Could you check a few things on this drawing? It's one solid part, dimensions in mm from its lowest x, y, z. Give positions to 0.01 mm unless a question says otherwise; leave off trailing zeros. Order: outer loops, then holes, each group sorted by start corner. A loop starts at its lowest first (then second) coordinate and runs counter-clockwise, first axis right, second up. Notation, with made-up numbers: (32.25, 26.25) -> (52.25, 26.25) arc R28 ccw to (52.25, 53.25) -> close; hole circle Ø3 at (72, 45.25). An arc over 180 degrees is marked (long way). Write each question's results on one line, items separated by ' | '. Start each with the question number.
Q1. I need wall thicknesses on line 1 along Z through (x, y) = (2.8, 5.25) (1 decimal); line 2 along Y through (x, z) = (0.9, 4) (1 decimal); line 3 along Y through (x, z) = (0.85, 10.75) (1 decimal). Which ranges of each line are inside material? Lowest first, please. Write a range as [from, to].
Q2. Imagine slicing it at C-C, the plane x = 2.25. Please give me the cut outline in (y, z), then the cut area to 3 significant figures.
Q3. Thinking about a two-plate mould opening in Z: for the marked faces 1, 2 and 3, which applies, pulls with the +Z half, pulls with the -Z half, needs draft (parallel to the pull), parting line crosses it, or undercut?
Q4. Imagine slicing it at D-D, the plane z = 3.5. Please give me the cut outline in (x, y).
Q5. Imagine slicing it at A-A, the plane y = 11. Please give me the cut outline in (x, z).
Q6. I'm going to push flat-ended pins straight in: pin 1 (1.8 mm diameter, centred on y = 17.01, z = 4.99, fed in from -X); pin 2 (1.5 mm diameter, centred on x = 1.5, z = 15, fed in from -Y). Where does each tip first touch, or does it pass through?
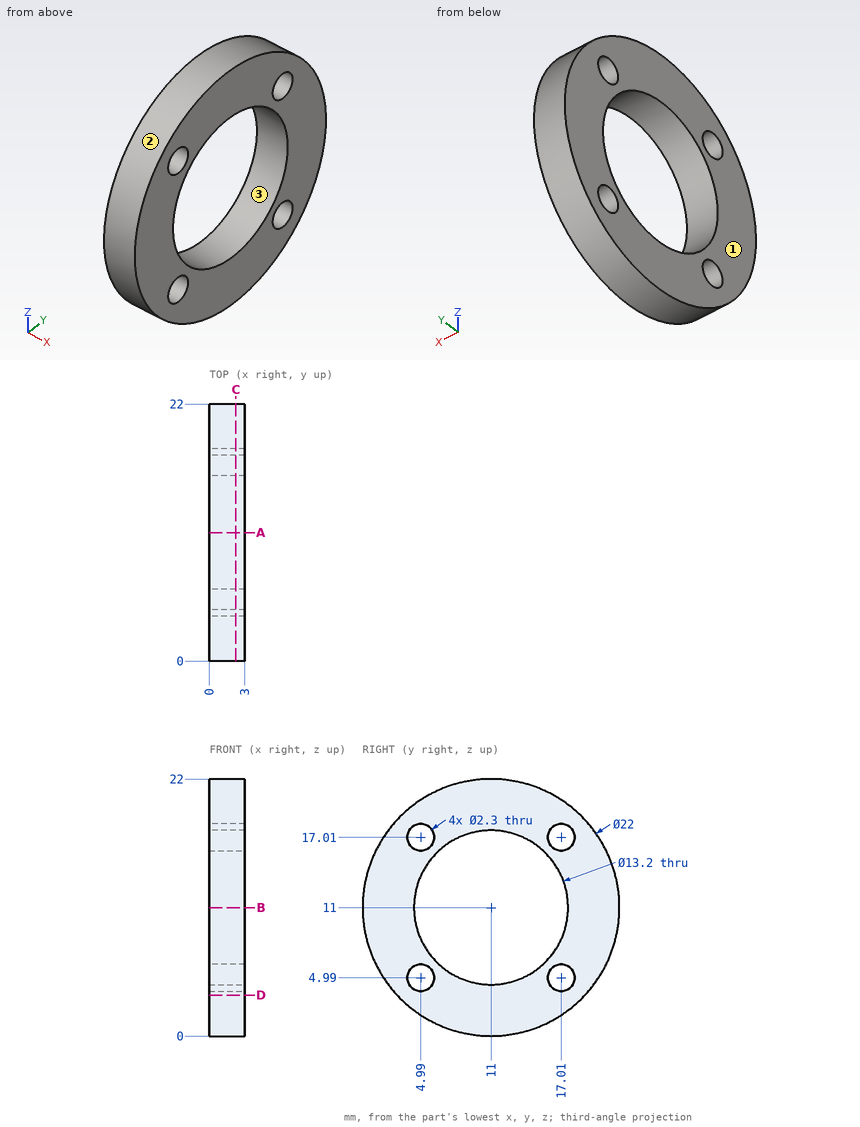
Geometry check:
1) line 1: [1.6, 3.9], [6.1, 7.8], [14.2, 15.9], [18.1, 20.4] | line 2: [2.5, 4.4], [5.6, 16.4], [17.6, 19.5] | line 3: [0, 4.4], [17.6, 22]
2) outline: circle Ø22 at (11, 11); hole circle Ø2.3 at (4.99, 4.99); hole circle Ø2.3 at (4.99, 17.01); hole circle Ø13.2 at (11, 11); hole circle Ø2.3 at (17.01, 4.99); hole circle Ø2.3 at (17.01, 17.01) | area: 227 mm²
3) face 1: needs draft | face 2: parting line crosses it | face 3: undercut
4) outline: (0, 2.95) -> (3, 2.95) -> (3, 19.05) -> (0, 19.05) -> close
5) outline: (0, 0) -> (3, 0) -> (3, 4.4) -> (0, 4.4) -> close; (0, 17.6) -> (3, 17.6) -> (3, 22) -> (0, 22) -> close
6) pin 1: through | pin 2: y = 0.49
